For this review, use the dimensioned drawing (mm, ordinates from the lowest corner) and the shaded views. A direction names the side the tool comes from. Round coordinates to 2 decimals unless told otherwise and drop trailing zeros. Order: outer loops, then holes, each group sorted by start corner. A loop starts at its lowest first (then second) coordinate and runs counter-clockwise, first axis right, second up. Notation, with made-up numbers: (50, 23.5) - (108, 23.5) arc R14 ccw to (108, 41.5) - close; hole circle Ø8 at (13, -37). An arc over 180 degrees is marked (long way). Write each question's results on one line, items separated by ' | '. Start each with the question number.
(1) For the marked faces 1, 2, 3 and 4, list the 3-axis set-ups (+Z, -Z, +X, -X, +Y, -Y) from which the entire face can be reached by the end or side of a thin tool; tool diameter is ignored.
(2) Take a section at D-D, the plane x = 165. Give the boundary of the cut face in (y, z).
(3) Draft analysis for pull direction Z (two halves, no side actions). For the marked faces 5, 6 and 7, state which applies: pulls with the +Z half, pulls with the -Z half, needs draft (parallel to the pull), parting line crosses it, or undercut.
(4) For L1, parallel to X at y = 55.5, z = 28.5; L2, parallel to X at y = 71.5, z = 63; L3, parallel to Z at x = 144, y = 39, list the stretches that pass through material, from the lowest coordinate up. Write a range as from..to.
(5) Take a section at B-B, the plane z = 8. Give the boundary of the cut face in (x, y), plus the area to 3 significant figures.
(6) Take a section at A-A, the plane z = 40. Give the number of separate pieces and of enclosed holes in the cut face, plus the area to 3 significant figures.
(7) Insertion check: pin 1 Ø1.5 at (x, y) = (191.5, 47.5) entering from -Z; pin 2 Ø6 at (x, y) = (102.5, 50.5) entering from +Z; pin 3 Ø4 at (x, z) = (193, 36) entering from -Y; pin 4 Ø9 at (y, z) = (37, 36.5) entering from -X. Each pin has a flat end and moves straight along its axis. Give the tip position at first contact, or say it passes through.
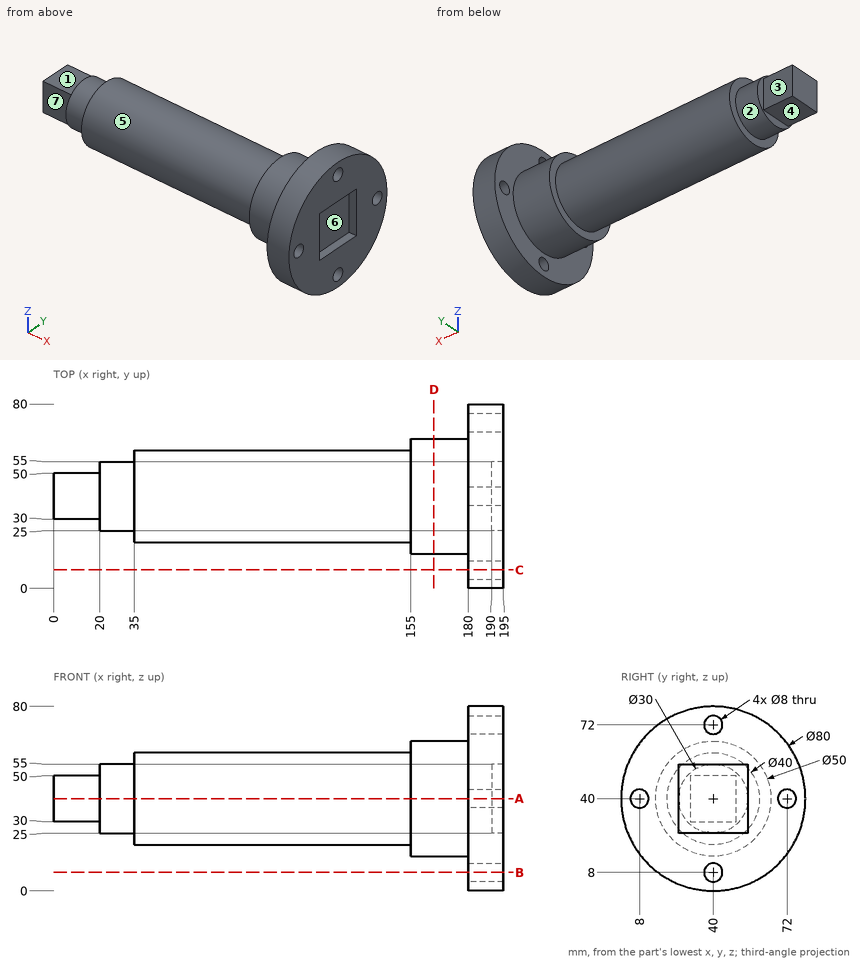
Results below:
1) face 1: +Z, -X, +Y, -Y | face 2: -X | face 3: +Z, -Z, -X, +Y | face 4: -Z, -X, +Y, -Y
2) outline: circle Ø50 at (40, 40)
3) face 5: parting line crosses it | face 6: undercut | face 7: needs draft
4) L1: x = 35..195 | L2: x = 180..195 | L3: z = 20.03..59.97
5) outline: (180, 16) - (195, 16) - (195, 36) - (180, 36) - close; (180, 44) - (195, 44) - (195, 64) - (180, 64) - close | area: 600 mm^2
6) separate pieces: 3 | enclosed holes: 0 | area: 7,710 mm^2
7) pin 1: stops at z = 0.57 | pin 2: stops at z = 58.54 | pin 3: stops at y = 0.05 | pin 4: stops at x = 0
